from build123d import *

# Parameters (mm, degrees)
F0_R          = 10
F0_R_2        = 4
F1_DEPTH      = 15
F2_R          = 0.5
F4_DEPTH      = 10
F4_DEPTH_BACK = 10


with BuildPart() as f1:
    # F0 (on Front) → F1 (new body)
    with BuildSketch(Plane.XZ):
        Circle(F0_R)
        Circle(F0_R_2, mode=Mode.SUBTRACT)
    extrude(amount=F1_DEPTH)

    # F2
    f2_edges = [f1.edges().sort_by_distance(p)[0] for p in [
        (-10, -15, 0),
        (-4, -15, 0),
    ]]
    fillet(f2_edges, radius=F2_R)

    # F3 (on Top) → F4 (cut, two sides)
    with BuildSketch(Plane.XY) as f4_sk:
        Polygon((10, 0), (-10, 0), (10, -5.358984), align=None)
    extrude(amount=F4_DEPTH, mode=Mode.SUBTRACT)
    extrude(f4_sk.sketch, amount=-F4_DEPTH_BACK, mode=Mode.SUBTRACT)


solid = f1.part
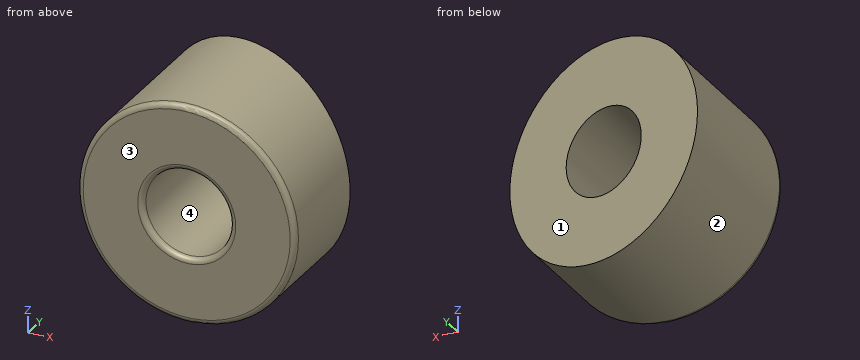
Check sheet for the modelled part. Datum: model origin and axes. Units: mm. Face numbers are marked on the shaded views. Give positions to 0.01 mm unless a question says otherwise; leave off trailing zeros. Order: outer loops, then holes, each group sorted by start corner. A loop starts at its lowest first (then second) coordinate and runs counter-clockwise, first axis right, second up. Notation, with made-up numbers: M 19,33.5 L 28,33.5 A17 cw 28,54.5 Z; hole C -2,66 d8. An arc over 180 degrees is marked long. Answer as CSV lines item,"result". Start each with the question number.
Item 1: Cross-section at C-C on y = -14. Enter the section's corners in (x, z).
Item 2: Gauge pin test, flat ends, axial feed: P1, Ø1, axis at y = -7, z = -5.5, coming from the +X side; P2, Ø4, axis at x = 5, z = -6, coming from the +Y side; P3, Ø4, axis at x = 4, y = -9.5, coming from the +Z side. Record the tip position at first contact, or that the pin passes through.
Item 3: Thickness scan on line 1 (Z direction, x = 0, y = -8.5); line 2 (Z direction, x = 3.5, y = -10.25). Record the ranges inside material, lowest first. Write a range as [from, to].
Item 4: Cross-section at B-B on x = 0. Enter the section's corners in (y, z).
Item 5: Mould release check, pull along X, two halves, no side actions. Record for the marked faces 1, 2, 3 and 4: +X half, -X half, draft (parallel to the pull), parting line (faces both ways), or undercut.
Item 6: Cross-section at A-A on z = 0. Enter the section's corners in (x, y).
Established:
1,outline,"C 0,0 d20; hole C 0,0 d8"
2,P1,"stops at x = 8.66"
2,P2,"stops at y = -3.48"
2,P3,"stops at z = 9.8"
3,line 1,"z = [-10, -4], [4, 10]"
3,line 2,"z = [-9.37, -1.94], [1.94, 9.37]"
4,outline,"M -15,-9.5 A0.5 ccw -14.5,-10 L -2.68,-10 L -2.68,-4 L -14.5,-4 A0.5 ccw -15,-4.5 Z; M -15,4.5 A0.5 ccw -14.5,4 L -2.68,4 L -2.68,10 L -14.5,10 A0.5 ccw -15,9.5 Z"
5,face 1,"+X half"
5,face 2,"parting line"
5,face 3,"draft"
5,face 4,"undercut"
6,outline,"M -10,-14.5 A0.5 ccw -9.5,-15 L -4.5,-15 A0.5 ccw -4,-14.5 L -4,-1.61 L -10,0 Z; M 4,-14.5 A0.5 ccw 4.5,-15 L 9.5,-15 A0.5 ccw 10,-14.5 L 10,-5.36 L 4,-3.75 Z"
